Input: part model. Units: mm. Frame: model coordinates. Give positions to 0.01 mm unless a question says otherwise; leave off trailing zeros. Write each loop counter-clockwise with the first axis right and the second up, starting at its lowest first coordinate (ties: lowest second). Pieces come first, ordered by that corner, then holes. Notation, with made-up numbers: (-12, -13.75) -> (44, -13.75) arc R26 ccw to (44, 24.25) -> close; hole circle Ø5 at (44, 12). An arc over 180 degrees is marked (long way). Return JSON: item names as keys, results as strings. Group by question number.
Item 1: Pin query (flat end, axial travel): P1, Ø5, axis at x = 31.5, z = 28.5, coming from the -Y side; P2, Ø4, axis at y = 375, z = 58.5, coming from the -X side; P3, Ø5.5, axis at x = 26, y = 192, coming from the +Z side; P4, Ø10, axis at x = 32, z = 156.5, coming from the -Y side. Return the tip coordinate at first contact, or that it passes through.
Item 2: Section B-B, the plane z = 143.5. Return loops of the section in (x, y).
Item 3: Section A-A, the plane y = 238.5. Return loops of the section in (x, z).
Item 4: Line query: line 1 (Z direction, x = 27.5, y = 248); line 2 (Z direction, x = 36, y = 210); line 3 (Y direction, x = 32, z = 190). Output: solid intervals per line, ascending. Write a range as [from, to].
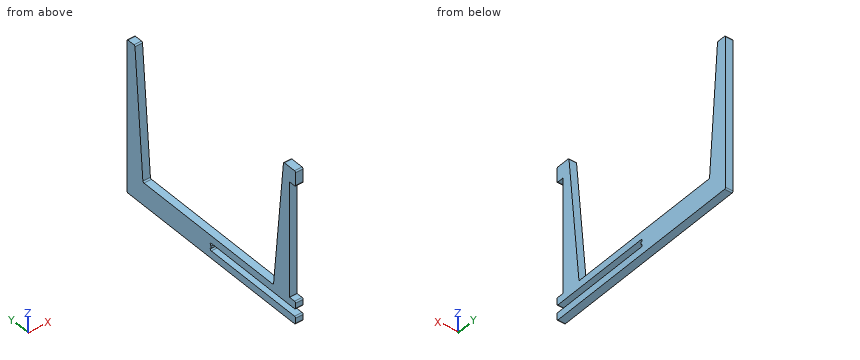
from build123d import *

# Parameters (mm, degrees)
F2_DEPTH = 19.05
F3_R     = 3.175
F5_DEPTH = 19.05
F6_R     = 3.175


with BuildPart() as f2:
    # F1 (on offset) → F2 (new body)
    with BuildSketch(Plane.YZ.offset(19.05)):
        Polygon((-19.05, 19.05), (-19.05, 0), (514.35, 0), (514.35, 387.35), (488.95, 387.35), (463.55, 57.15), (50.8, 57.15), (19.05, 387.35), (-19.05, 387.35), (-19.05, 349.25), (0, 349.25), (0, 57.15), (-19.05, 57.15), (-19.05, 38.1), (247.65, 38.1), (247.65, 19.05), align=None)
    extrude(amount=F2_DEPTH)

    # F3
    f3_edges = [f2.edges().sort_by_distance(p)[0] for p in [
        (28.575, -19.05, 0),
        (28.575, -19.05, 19.05),
        (28.575, -19.05, 38.1),
        (28.575, -19.05, 57.15),
        (28.575, -19.05, 349.25),
        (28.575, -19.05, 387.35),
        (28.575, 19.05, 387.35),
        (28.575, 50.8, 57.15),
        (28.575, 463.55, 57.15),
        (28.575, 488.95, 387.35),
    ]]
    fillet(f3_edges, radius=F3_R)

    # F4 (on face) → F5 (cut)
    with BuildSketch(Plane.YZ.offset(38.1)):
        with BuildLine():
            Line((247.65, 25.4), (247.65, 19.05))
            ThreePointArc((247.65, 19.05), (250.825, 22.225), (247.65, 25.4))
        make_face()
        with BuildLine():
            ThreePointArc((247.65, 31.75), (250.825, 34.925), (247.65, 38.1))
            Line((247.65, 38.1), (247.65, 31.75))
        make_face()
    extrude(amount=-F5_DEPTH, mode=Mode.SUBTRACT)

    # F6
    f6_edges = [f2.edges().sort_by_distance(p)[0] for p in [
        (28.575, 514.35, 0),
        (28.575, 514.35, 387.35),
    ]]
    fillet(f6_edges, radius=F6_R)


solid = f2.part
Answer below:
{
 "1": {"P1": "stops at y = 247.65", "P2": "stops at x = 19.05", "P3": "stops at z = 57.15", "P4": "stops at y = 0"},
 "2": {"outline": "(19.05, 0) -> (38.1, 0) -> (38.1, 42.5) -> (19.05, 42.5) -> close; (19.05, 470.19) -> (38.1, 470.19) -> (38.1, 514.35) -> (19.05, 514.35) -> close"},
 "3": {"outline": "(19.05, 0) -> (38.1, 0) -> (38.1, 19.05) -> (19.05, 19.05) -> close; (19.05, 38.1) -> (38.1, 38.1) -> (38.1, 57.15) -> (19.05, 57.15) -> close"},
 "4": {"line 1": "z = [0, 19.07], [25.38, 31.77], [38.08, 57.15]", "line 2": "z = [0, 19.05], [38.1, 57.15]", "line 3": "y = [0, 38.03], [473.77, 514.35]"}
}
